Design review of the part built by this model. Coordinates are the model's own, in mm. Face numbers are marked on the shaded views. A direction names the side the tool comes from. Give positions to 0.01 mm unless a question says otherwise; leave off trailing zeros. Loops run counter-clockwise (first coordinate to the right, second up) from the corner with the lowest first, then second, coordinate; pieces in that order, holes last. Notation, with made-up numbers: M -22,11.25 L 29,11.25 A22 ccw 29,44.25 Z; hole C 59.5,47.25 d8. An arc over 180 degrees is marked long. Use one line per item in the form item = value. Start each with the question number.
from build123d import *

# Parameters (mm, degrees)
SKETCH1_W                    = 74
SKETCH1_H                    = 74.2
BOSS_EXTRUDE1_DEPTH          = 15.425
SKETCH3_W                    = 8
SKETCH3_H                    = 21.5
CUT_EXTRUDE1_DEPTH           = 26.1
F_30_0_1285_DIAMETER_HOLE1_D = 3.2639
SKETCH6_W                    = 31
SKETCH6_H                    = 20
BOSS_EXTRUDE2_DEPTH          = 2
SKETCH7_R                    = 2
BOSS_EXTRUDE3_DEPTH          = 20


with BuildPart() as part:
    # Sketch1 → Boss-Extrude1 (new, symmetric)
    with BuildSketch(Plane(origin=(0, 0, 0), x_dir=(1, 0, 0), z_dir=(0, 1, 0))):
        Rectangle(SKETCH1_W, SKETCH1_H)
    extrude(amount=BOSS_EXTRUDE1_DEPTH, both=True)

    # Sketch3 → Cut-Extrude1 (cut)
    with BuildSketch(Plane(origin=(0, 15.425, 0), x_dir=(1, 0, 0), z_dir=(0, 1, 0))):
        with Locations((-33, 0)):
            Rectangle(SKETCH3_W, SKETCH3_H)
    cut_extrude1 = extrude(amount=-CUT_EXTRUDE1_DEPTH, mode=Mode.SUBTRACT)

    # #30 (0.1285) Diameter Hole1 (through all)
    with Locations(Plane(origin=(0, -10.675, 0), x_dir=(1, 0, 0), z_dir=(0, 1, 0))):
        with Locations((-33, 0)):
            f_30_0_1285_diameter_hole1 = Hole(F_30_0_1285_DIAMETER_HOLE1_D / 2)

    # Sketch6 → Boss-Extrude2 (add)
    with BuildSketch(Plane.XY.offset(37.1)):
        with Locations((0, -5.425)):
            Rectangle(SKETCH6_W, SKETCH6_H)
    extrude(amount=BOSS_EXTRUDE2_DEPTH)

    # Sketch7 → Boss-Extrude3 (add)
    with BuildSketch(Plane.XY.offset(39.1)):
        with Locations((-9, -5.425)):
            Circle(SKETCH7_R)
        with Locations((-3, -5.425)):
            Circle(SKETCH7_R)
    boss_extrude3 = extrude(amount=BOSS_EXTRUDE3_DEPTH)

    # Mirror1: Cut-Extrude1, #30 (0.1285) Diameter Hole1, Boss-Extrude3 across plane
    add(cut_extrude1.mirror(Plane(origin=(0, 0, 0), x_dir=(0, 0, 1), z_dir=(1, 0, 0))), mode=Mode.SUBTRACT)
    add(f_30_0_1285_diameter_hole1.mirror(Plane(origin=(0, 0, 0), x_dir=(0, 0, 1), z_dir=(1, 0, 0))), mode=Mode.SUBTRACT)
    add(boss_extrude3.mirror(Plane(origin=(0, 0, 0), x_dir=(0, 0, 1), z_dir=(1, 0, 0))))


solid = part.part
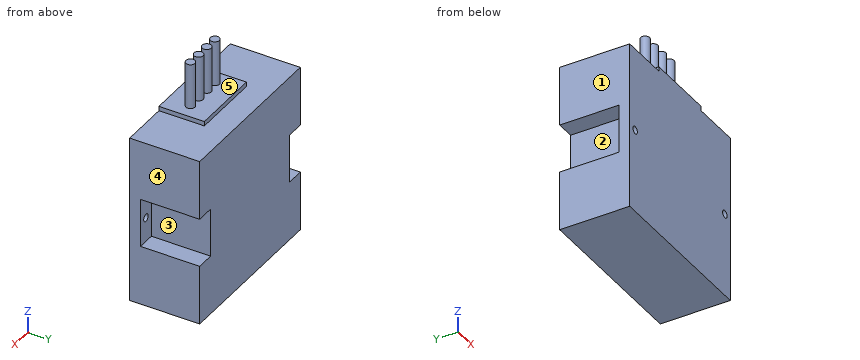
Q1. Clearance check with flat-ended pins moving along their axes: pin 1 Ø2 at (x, z) = (-33, 0) entering from +Y; pin 2 Ø9 at (x, z) = (-34.5, -3) entering from +Y (3 decimals); pin 3 Ø1 at (y, z) = (-9.5, 38) entering from -X; pin 4 Ø8 at (x, y) = (5.5, -9) entering from +Z. State where each tip first meets the part, or that it passes through.
Q2. Take a section at D-D on x = 9. Give the boundary of the cut face in (y, z) (3 decimals), plus the area to 3 significant figures.
Q3. Take a section at A-A on z = 0. Give the boundary of the cut face in (x, y) (3 decimals), plus the area to 3 significant figures.
Q4. Take a section at C-C on y = 13. Give the boundary of the cut face in (x, z), plus the area to 3 significant figures.
Q5. Take a section at B-B on x = 33. Give the boundary of the cut face in (y, z) (3 decimals).
Q6. The part is to be moulded in two halves that separate along Z. For the marked faces 3, 4 and 5, say which applies: pulls with the +Z half, pulls with the -Z half, needs draft (parallel to the pull), parting line crosses it, or undercut.
Q7. For the marked faces 1 and 2, list the 3-axis set-ups (+Z, -Z, +X, -X, +Y, -Y) from which the entire face can be reached by the end or side of a thin tool; tool diameter is ignored.
Q8. Wall thickness on probe 1 along Z at (x, y) = (-33, -14); probe 2 along Z at (x, y) = (32, -4); probe 3 along Z at (x, y) = (-2, -2): over which ranges is each line inside the solid? List them lowest first.
Response values:
q1.pin_1 = through
q1.pin_2 = -10.675
q1.pin_3 = -15.5
q1.pin_4 = 59.1
q2.outline = M -15.425,-37.1 L 15.425,-37.1 L 15.425,37.1 L 4.575,37.1 L 4.575,39.1 L -3.425,39.1 L -3.425,59.1 L -7.425,59.1 L -7.425,39.1 L -15.425,39.1 Z
q2.area = 2,410 mm^2
q3.outline = M -37,-15.425 L -34.632,-15.425 L -34.632,-10.675 L -37,-10.675 Z; M -31.368,-15.425 L 31.368,-15.425 L 31.368,-10.675 L 29,-10.675 L 29,15.425 L -29,15.425 L -29,-10.675 L -31.368,-10.675 Z; M 34.632,-15.425 L 37,-15.425 L 37,-10.675 L 34.632,-10.675 Z
q3.area = 1,830 mm^2
q4.outline = M -37,-37.1 L 37,-37.1 L 37,-10.75 L 29,-10.75 L 29,10.75 L 37,10.75 L 37,37.1 L -37,37.1 L -37,10.75 L -29,10.75 L -29,-10.75 L -37,-10.75 Z
q4.area = 5,150 mm^2
q5.outline = M -15.425,-37.1 L 15.425,-37.1 L 15.425,-10.75 L -10.675,-10.75 L -10.675,-1.632 L -15.425,-1.632 Z; M -15.425,1.632 L -10.675,1.632 L -10.675,10.75 L 15.425,10.75 L 15.425,37.1 L -15.425,37.1 Z
q6.face_3 = undercut
q6.face_4 = needs draft
q6.face_5 = pulls with the +Z half
q7.face_1 = +Z, -Z, -X, +Y, -Y
q7.face_2 = -X, +Y
q8.probe_1 = -37.1 to -1.63, 1.63 to 37.1
q8.probe_2 = -37.1 to -10.75, 10.75 to 37.1
q8.probe_3 = -37.1 to 39.1
